The model under review builds one solid part; all positions refer to its coordinate system, in mm. A direction names the side the tool comes from. Coordinates: 2 decimals unless noted, no trailing zeros. Order: outer loops, then holes, each group sorted by start corner. A loop starts at its lowest first (then second) coordinate and runs counter-clockwise, first axis right, second up.
Autodesk Inventor part; units mm, degrees
ref_plane "YZ Plane" through (0, 0, 0) normal (1, 0, 0) x (0, 1, 0)
ref_plane "XZ Plane" through (0, 0, 0) normal (0, 1, 0) x (-1, 0, 0)
ref_plane "XY Plane" through (0, 0, 0) normal (0, 0, 1) x (1, 0, 0)
sketch "Sketch1" plane through (0, 0, 0) normal (0, 1, 0) x (-1, 0, 0)
  line L0 (37.5, -25) -> (-37.5, -25) construction
  line L1 (-37.5, -25) -> (-37.5, 25) construction
  line L2 (-37.5, 25) -> (37.5, 25) construction
  line L3 (37.5, 25) -> (37.5, -25) construction
  arc A0 (6.8822, -25) -> (6.8822, 25) centre (0, 0) ccw
  arc A1 (-6.8822, 25) -> (-6.8822, -25) centre (0, 0) ccw
  line L4 (6.8822, -25) -> (-6.8822, -25)
  line L5 (-6.8822, 25) -> (6.8822, 25)
  dimension "d4" = 50
  dimension "d5" = 75
extrude "Extrusion1" add sketch "Sketch1" along normal blind 12.65
sketch "Sketch2" plane through (0, 12.65, 0) normal (0, 1, 0) x (1, 0, 0)
  line L0 (-37.5, 25) -> (37.5, 25) construction
  line L1 (-37.5, -25) -> (-37.5, 25) construction
  line L2 (37.5, 25) -> (37.5, -25) construction
  line L3 (37.5, -25) -> (-37.5, -25) construction
  line L4 (-37.5, 25) -> (37.5, 25)
  line L5 (37.5, -25) -> (37.5, 25)
  line L6 (37.5, -25) -> (-37.5, -25)
  line L7 (-37.5, -25) -> (-37.5, 25)
  point P0 (0, 0)
extrude "Extrusion2" add sketch "Sketch2" along normal blind 1
sketch "Sketch3" plane through (0, 13.65, 0) normal (0, 1, 0) x (1, 0, 0)
  line L0 (37.5, -25) -> (6.8822, -25)
  line L1 (12.8, -25) -> (12.8, 25)
  line L2 (12.8, 25) -> (37.5, 25)
  line L3 (37.5, -25) -> (37.5, 25)
  line L4 (37.5, 25) -> (37.5, -25)
  line L5 (37.5, -25) -> (12.8, -25)
  line L6 (-12.8, -25) -> (-12.8, 25)
  line L7 (-37.5, 25) -> (-37.5, -25)
  line L8 (-12.8, 25) -> (-37.5, 25)
  line L9 (-37.5, 25) -> (-37.5, -25)
  line L10 (-37.5, -25) -> (-12.8, -25)
  point P0 (0, 0)
  dimension "d12" = 25.6
  dimension "d13" = 24.7
  dimension "d14" = 24.7
extrude "Extrusion3" add sketch "Sketch3" along normal blind 12.4 contours L10 L7 L8 L6
extrude "Extrusion4" add sketch "Sketch3" along normal blind 12.45 contours L0 L1 L2 L3
sketch "Sketch4" plane through (0, 13.65, 0) normal (0, 1, 0) x (1, 0, 0)
  circle A0 centre (0, 21.91) radius 1.5
  circle A1 centre (0, -21.91) radius 1.5
  circle A2 centre (0, 1.95) radius 1.5
  line L0 (12.8, 25) -> (12.8, -25)
  point P0 (0, 0)
  dimension "d21" = 3
  dimension "d23" = 3
  dimension "d25" = 3
  dimension "d26" = 21.91
  dimension "d27" = 23.86
  dimension "d28" = 21.91
  dimension "d29" = 12.8
extrude "Extrusion5" cut sketch "Sketch4" against normal blind 18.8
sketch "Sketch5" plane through (0, 26.05, 0) normal (0, 1, 0) x (1, 0, 0)
  circle A0 centre (-29.4, 12.15) radius 1.5
  circle A1 centre (-29.4, -12.15) radius 1.5
  circle A2 centre (-31.8, 0) radius 2.2
  line L0 (-37.5, 25) -> (-37.5, -25)
  circle A3 centre (29.4, 12.15) radius 1.5
  circle A4 centre (29.4, -12.15) radius 1.5
  circle A5 centre (31.8, 0) radius 2.2
  circle A6 centre (29.4, 12.15) radius 1.5
  circle A7 centre (29.4, -12.15) radius 1.5
  circle A8 centre (31.8, 0) radius 2.2
  point P0 (0, 0)
  dimension "d35" = 3
  dimension "d36" = 3
  dimension "d37" = 4.4
  dimension "d38" = 8.1
  dimension "d41" = 5.7
extrude "Extrusion6" cut sketch "Sketch5" along normal mid plane 35
sketch "Sketch7" plane through (0, 26.1, 0) normal (0, 1, 0) x (1, 0, 0)
  circle A0 centre (31.8, 0) radius 3.7
  point P0 (0, 0)
  dimension "d44" = 7.4
extrude "Extrusion7" cut sketch "Sketch7" against normal blind 5
sketch "Sketch8" plane through (0, 26.05, 0) normal (0, 1, 0) x (1, 0, 0)
  circle A0 centre (-31.8, 0) radius 3.7
  point P0 (0, 0)
  dimension "d47" = 7.4
extrude "Extrusion8" cut sketch "Sketch8" against normal blind 5
properties part number "PocketNC_Vise_Backing_Plate" material "Aluminum 6061"
(1) Machinability: for faces 5 (the face through (-12.8, 20, 0)), 6 (the face through (29, 12.65, 0)), 7 (the face through (-25.926, 6.236, 0.473)), 8 (the face through (28.104, 23.635, -0.163)), which of the approach directions +Z, -Z, +X, -X, +Y, -Y give a long, thin tool a straight path to every point of the face, cutting with its end or side? Answer none if there is none.
A:
face 5: +Z, -Z, +Y
face 6: +X, -Y
face 7: -X, -Y
face 8: +Y
(2) Draft analysis for pull direction X (two halves, no side actions). For faces 1 (the face through (25.926, 6.236, -0.473)), 2 (the face through (30.83, 19.47, -12.6)), 3 (the face through (-25, 26.05, 0)), 4 (the face through (31.7, 21.1, 2.4)), state which applies: released by +X, released by -X, zero draft, split by the parting line, or undercut.
A:
face 1: released by +X
face 2: undercut
face 3: zero draft
face 4: undercut
(3) Wall thickness on probe 1 along Z at (x, y) = (0, 9.25); probe 2 along X at (y, z) = (17.25, -12.15); probe 3 along X at (y, z) = (24.85, 0): over which ranges is each line inside the solid? List them lowest first.
A:
probe 1: z = -25 to -23.41, -20.41 to -3.45, -0.45 to 20.41, 23.41 to 25
probe 2: x = -37.5 to -30.9, -27.9 to -12.8, 12.8 to 27.9, 30.9 to 37.5
probe 3: x = -37.5 to -35.5, -28.1 to -12.8, 12.8 to 28.1, 35.5 to 37.5
(4) We need section C-C, the plane x = 0. Write out the cut boundary in (y, z).
A:
outline: (0, -25) - (13.65, -25) - (13.65, -23.41) - (0, -23.41) - close; (0, -20.41) - (13.65, -20.41) - (13.65, -3.45) - (0, -3.45) - close; (0, -0.45) - (13.65, -0.45) - (13.65, 20.41) - (0, 20.41) - close; (0, 23.41) - (13.65, 23.41) - (13.65, 25) - (0, 25) - close
(5) For pin 1 Ø4.5 at (x, z) = (31.8, 0) entering from -Y; pin 2 Ø8 at (x, z) = (-31.5, 1) entering from +Y; pin 3 Ø3.5 at (x, z) = (33, 0.5) entering from +Y, all flat-tipped, find the tip position at first contact; note any pin that passes through.
A:
pin 1: stops at y = 12.65
pin 2: stops at y = 26.05
pin 3: stops at y = 21.1
(6) We need section A-A, the plane x = 31.8. Write out the cut boundary in (y, z), and give its area (3 significant figures).
A:
outline: (12.65, -25) - (26.1, -25) - (26.1, -3.7) - (21.1, -3.7) - (21.1, -2.2) - (12.65, -2.2) - close; (12.65, 2.2) - (21.1, 2.2) - (21.1, 3.7) - (26.1, 3.7) - (26.1, 25) - (12.65, 25) - close
area: 598 mm2
(7) We need section D-D, the plane z = 12.15. Write out the cut boundary in (x, y).
A:
outline: (-37.5, 12.65) - (-30.9, 12.65) - (-30.9, 26.05) - (-37.5, 26.05) - close; (-27.9, 12.65) - (-22.91, 12.65) - (-22.91, 0) - (22.91, 0) - (22.91, 12.65) - (27.9, 12.65) - (27.9, 26.1) - (12.8, 26.1) - (12.8, 13.65) - (-12.8, 13.65) - (-12.8, 26.05) - (-27.9, 26.05) - close; (30.9, 12.65) - (37.5, 12.65) - (37.5, 26.1) - (30.9, 26.1) - close
(8) We need section B-B, the plane y = 16. Write out the cut boundary in (x, z), and give its area (3 significant figures).
A:
outline: (-37.5, -25) - (-12.8, -25) - (-12.8, 25) - (-37.5, 25) - close; (12.8, -25) - (37.5, -25) - (37.5, 25) - (12.8, 25) - close; hole circle Ø4.4 at (-31.8, 0); hole circle Ø3 at (-29.4, -12.15); hole circle Ø3 at (-29.4, 12.15); hole circle Ø3 at (29.4, -12.15); hole circle Ø3 at (29.4, 12.15); hole circle Ø4.4 at (31.8, 0)
area: 2,410 mm2
